```python
from build123d import *

# Parameters (mm, degrees)
F1_DEPTH = 38.1
F2_DEPTH = 38.1
F3_R     = 6.35
F4_DEPTH = 38.1
F5_R     = 6.35
F6_DEPTH = 38.1


with BuildPart() as f1:
    # F0 (on Front) → F1 (new body)
    with BuildSketch(Plane.XZ):
        Polygon((323.85, 635), (-285.75, 635), (-285.75, 596.9), (0, 596.9), (0, 165.1), (-114.3, 165.1), (-114.3, 127), (0, 127), (0, 0), (38.1, 0), (38.1, 127), (152.4, 127), (152.4, 165.1), (38.1, 165.1), (38.1, 596.9), (323.85, 596.9), align=None)
    extrude(amount=F1_DEPTH)

    # F0 (on Front) → F2 (join)
    with BuildSketch(Plane.XZ):
        Polygon((323.85, 635), (-285.75, 635), (-285.75, 596.9), (0, 596.9), (0, 165.1), (-114.3, 165.1), (-114.3, 127), (0, 127), (0, 0), (38.1, 0), (38.1, 127), (152.4, 127), (152.4, 165.1), (38.1, 165.1), (38.1, 596.9), (323.85, 596.9), align=None)
    extrude(amount=F2_DEPTH)

    # F3 (on face) → F4 (join)
    with BuildSketch(Plane.XZ.offset(38.1)):
        with Locations((-234.95, 615.95)):
            Circle(F3_R)
        with Locations((-110.49, 615.95)):
            Circle(F3_R)
        with Locations((19.05, 615.95)):
            Circle(F3_R)
        with Locations((148.59, 615.95)):
            Circle(F3_R)
        with Locations((273.05, 615.93546)):
            Circle(F3_R)
        with Locations((-63.5, 146.05)):
            Circle(F3_R)
        with Locations((101.6, 146.05)):
            Circle(F3_R)
    extrude(amount=F4_DEPTH)

    # F5 (on face) → F6 (cut)
    with BuildSketch(Plane.XZ.offset(38.1)):
        with Locations((19.05, 439.42)):
            Circle(F5_R)
        with Locations((19.05, 243.84)):
            Circle(F5_R)
        with Locations((19.05, 48.26)):
            Circle(F5_R)
    extrude(amount=-F6_DEPTH, mode=Mode.SUBTRACT)


solid = f1.part
```
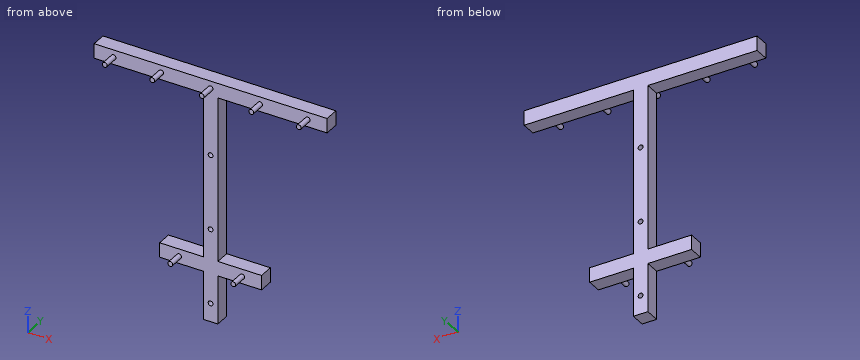
The model under review builds one solid part; all positions refer to its coordinate system, in mm. Give positions to 0.01 mm unless a question says otherwise; leave off trailing zeros. Loops run counter-clockwise (first coordinate to the right, second up) from the corner with the lowest first, then second, coordinate; pieces in that order, holes last. Notation, with made-up numbers: (36, 36.5) -> (80, 36.5) arc R24 ccw to (80, 72.5) -> close; hole circle Ø8 at (-1.5, 5). An arc over 180 degrees is marked (long way). Use CSV: the item, a comma, the result in double quotes.
1. For P1, Ø19, axis at y = -20.5, z = 72.5, coming from the +X side; P2, Ø19, axis at x = 148.5, y = -16, coming from the -Z side; P3, Ø6, axis at x = 156.5, y = -63, coming from the +Z side; P4, Ø11.5, axis at x = 19.05, z = 439.42, coming from the +Y side, all flat-tipped, find the tip position at first contact; note any pin that passes through.
Result:
P1,"stops at x = 38.1"
P2,"stops at z = 127"
P3,"stops at z = 619.98"
P4,"passes through"
2. Consider section A-A, the plane x = 46. Write out the cut boundary in (y, z).
Result:
outline,"(-38.1, 127) -> (0, 127) -> (0, 165.1) -> (-38.1, 165.1) -> close; (-38.1, 596.9) -> (0, 596.9) -> (0, 635) -> (-38.1, 635) -> close"
3. Consider section B-B, the plane y = -22. Write out the cut boundary in (x, z).
Result:
outline,"(-285.75, 596.9) -> (0, 596.9) -> (0, 165.1) -> (-114.3, 165.1) -> (-114.3, 127) -> (0, 127) -> (0, 0) -> (38.1, 0) -> (38.1, 127) -> (152.4, 127) -> (152.4, 165.1) -> (38.1, 165.1) -> (38.1, 596.9) -> (323.85, 596.9) -> (323.85, 635) -> (-285.75, 635) -> close; hole circle Ø12.7 at (19.05, 48.26); hole circle Ø12.7 at (19.05, 243.84); hole circle Ø12.7 at (19.05, 439.42)"
4. Consider section C-C, the plane y = -58. Write out the cut boundary in (x, z).
Result:
outline,"circle Ø12.7 at (-234.95, 615.95); circle Ø12.7 at (-110.49, 615.95); circle Ø12.7 at (-63.5, 146.05); circle Ø12.7 at (19.05, 615.95); circle Ø12.7 at (101.6, 146.05); circle Ø12.7 at (148.59, 615.95); circle Ø12.7 at (273.05, 615.94)"
5. Consider section D-D, the plane z = 576.5. Write out the cut boundary in (x, y).
Result:
outline,"(0, -38.1) -> (38.1, -38.1) -> (38.1, 0) -> (0, 0) -> close"
6. To check wall thickness, follow probe 1 along Z at (x, y) = (19.05, -10.5); probe 2 along Z at (x, y) = (112, -27); probe 3 along X at (y, z) = (-15.5, 439.42). State the ranges of each line that lie inside material, in increasing order. Write a range as from..to.
Result:
probe 1,"z = 0..41.91, 54.61..237.49, 250.19..433.07, 445.77..635"
probe 2,"z = 127..165.1, 596.9..635"
probe 3,"x = 0..12.7, 25.4..38.1"
